```python
from build123d import *

# Parameters (mm, degrees)
F1_DEPTH = 6
F3_D     = 5.1054
F3_DEPTH = 50.8


with BuildPart() as f1:
    # F0 (on Front) → F1 (new body)
    with BuildSketch(Plane.XZ):
        with BuildLine():
            ThreePointArc((-145.15302, 139.997129), (-147.398084, 139.067193), (-148.32802, 136.822129))
            Line((-148.32802, 136.822129), (-148.32802, 16.172129))
            ThreePointArc((-148.32802, 16.172129), (-147.398084, 13.927065), (-145.15302, 12.997129))
            Line((-145.15302, 12.997129), (-24.50302, 12.997129))
            ThreePointArc((-24.50302, 12.997129), (-22.257956, 13.927065), (-21.32802, 16.172129))
            Line((-21.32802, 16.172129), (-21.32802, 37.082001))
            ThreePointArc((-21.32802, 37.082001), (-21.569703, 38.297021), (-22.257956, 39.327065))
            Line((-22.257956, 39.327065), (-121.998084, 139.067193))
            ThreePointArc((-121.998084, 139.067193), (-123.028128, 139.755447), (-124.243148, 139.997129))
            Line((-124.243148, 139.997129), (-145.15302, 139.997129))
        make_face()
    extrude(amount=F1_DEPTH)

    # F3
    with Locations(Plane.XZ.offset(6)):
        with Locations((-135.62802, 76.497129), (-135.62802, 51.097129), (-135.62802, 25.697129), (-135.62802, 101.897129), (-135.62802, 127.297129), (-110.22802, 25.697129), (-84.82802, 25.697129), (-59.42802, 25.697129), (-34.02802, 25.697129)):
            Hole(F3_D / 2, depth=F3_DEPTH)


solid = f1.part
```
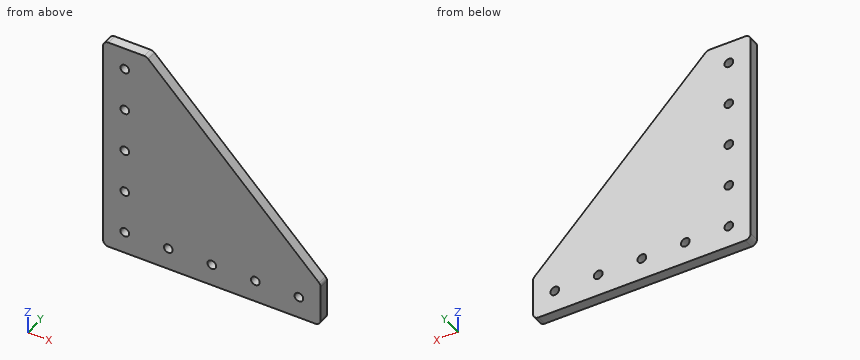
Can you work these out from the model? Positions are in its coordinate system, mm. Round coordinates to 2 decimals unless told otherwise and drop trailing zeros. Loops run counter-clockwise (first coordinate to the right, second up) from the corner with the lowest first, then second, coordinate; pieces in that order, holes last. Notation, with made-up numbers: (16, 75.25) -> (57, 75.25) arc R13 ccw to (57, 83.25) -> close; hole circle Ø3 at (45, -36.75). An arc over 180 degrees is marked (long way). One line per item, written item: value. Start each with the question number.
1. If we section it at B-B, the plane x = -33: Write out the boundary of the cut face in (y, z), then the cut area to 3 significant figures.
2. If I drill on probe 1 along X at (y, z) = (-2.8, 51.5); probe 2 along Z at (x, y) = (-36, -5.05); probe 3 along Z at (x, y) = (-59.5, -4.2), over which ranges is the centre line in solid material (lowest first)?
3. If we section it at D-D, the plane x = -66.5: Write out the boundary of the cut face in (y, z).
4. If we section it at C-C, the plane z = 112: Write out the boundary of the cut face in (x, y).
5. If we section it at A-A, the plane y = -4.7: Give the number of separate pieces and of enclosed holes in the cut face, then the cut area to 3 significant figures.
6. For pin 1 (2 mm diameter, centred on y = -3, z = 94.5, fed in from +X); pin 2 (4.5 mm diameter, centred on x = -84.83, z = 25.7, fed in from +Y); pin 3 (1.5 mm diameter, centred on y = -3.5, z = 98, fed in from +X), each with a flat end and sliding along its axis, tell me the tip position at first contact or that it passes through.
Calculated:
1. outline: (-6, 13) -> (0, 13) -> (0, 23.36) -> (-6, 23.36) -> close; (-6, 28.03) -> (0, 28.03) -> (0, 50.07) -> (-6, 50.07) -> close
1. area: 194 mm²
2. probe 1: x = -148.33 to -138.15, -133.11 to -34.43
2. probe 2: z = 13 to 24.08, 27.32 to 53.07
2. probe 3: z = 13 to 23.15, 28.25 to 76.57
3. outline: (-6, 13) -> (0, 13) -> (0, 83.57) -> (-6, 83.57) -> close
4. outline: (-148.33, -6) -> (-94.93, -6) -> (-94.93, 0) -> (-148.33, 0) -> close
5. separate pieces: 1
5. enclosed holes: 9
5. area: 10,800 mm²
6. pin 1: stops at x = -76.43
6. pin 2: passes through
6. pin 3: stops at x = -80.18
